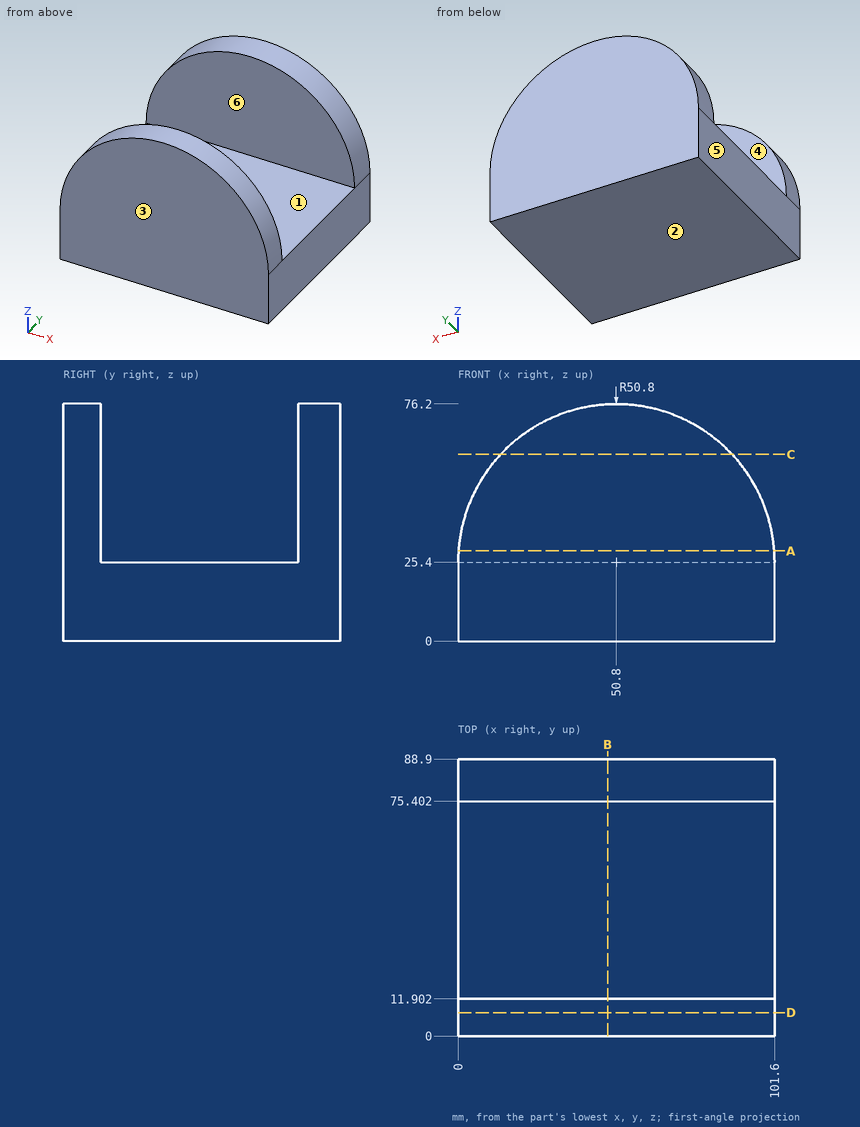
Geometry check sheet. Reference: drawing and pictorial views, mm from the part's lowest x, y, z. A direction names the side the tool comes from. Round coordinates to 2 decimals unless told otherwise and drop trailing zeros. Write each loop counter-clockwise with the first axis right and the second up, starting at its lowest first coordinate (ties: lowest second). Pieces come first, ordered by that corner, then holes.
1. Gauge pin test, flat ends, axial feed: P1, Ø15, axis at x = 51, z = 61, coming from the -Y side; P2, Ø4, axis at x = 19.5, y = 23.5, coming from the +Z side. Record the tip position at first contact, or that the pin passes through.
2. Section check C-C on z = 60. Enter the section's corners in (x, y), plus the area to 3 significant figures.
3. Section check B-B on x = 48. Enter the section's corners in (y, z).
4. Section check A-A on z = 29. Enter the section's corners in (x, y), plus the area to 3 significant figures.
5. Section check D-D on y = 7.5. Enter the section's corners in (x, z).
6. Scan lines: L1, parallel to Y at x = 69, z = 29.5; L2, parallel to Z at x = 86.5, y = 22.5; L3, parallel to Z at x = 9.5, y = 6. Record each from-to range of solid material in increasing order.
7. Access from +Z, -Z, +X, -X, +Y, -Y to the whole of each face (thin tool, end or side, straight path). Record for the marked faces 5 and 6.
8. Draft check along Y on the marked faces 1, 2, 3 and 4. Enter one of: +Y half, -Y half, draft (parallel to the pull), parting line (faces both ways), or undercut.
Answer:
1. P1: stops at y = 0
1. P2: stops at z = 25.4
2. outline: (13.6, 0) - (88, 0) - (88, 11.9) - (13.6, 11.9) - close; (13.6, 75.4) - (88, 75.4) - (88, 88.9) - (13.6, 88.9) - close
2. area: 1,890 mm2
3. outline: (0, 0) - (88.9, 0) - (88.9, 76.12) - (75.4, 76.12) - (75.4, 25.4) - (11.9, 25.4) - (11.9, 76.12) - (0, 76.12) - close
4. outline: (0.13, 0) - (101.47, 0) - (101.47, 11.9) - (0.13, 11.9) - close; (0.13, 75.4) - (101.47, 75.4) - (101.47, 88.9) - (0.13, 88.9) - close
4. area: 2,570 mm2
5. outline: (0, 0) - (101.6, 0) - (101.6, 25.4) arc R50.8 ccw to (0, 25.4) - close
6. L1: y = 0 to 11.9, 75.4 to 88.9
6. L2: z = 0 to 25.4
6. L3: z = 0 to 54.98
7. face 5: +Z, -Z, -X, +Y, -Y
7. face 6: +Z, +X, -X
8. face 1: undercut
8. face 2: draft
8. face 3: -Y half
8. face 4: undercut
